Here's how the part is built. I have some questions about the finished solid (model axes, mm). Coordinates: 2 decimals unless noted, no trailing zeros. Loops run counter-clockwise (first coordinate to the right, second up) from the corner with the lowest first, then second, coordinate; pieces in that order, holes last. Notation, with made-up numbers: M 27.25,49.25 L 43.25,49.25 A24 ccw 43.25,88.25 Z; hole C -22.75,52.25 d11. An arc over 180 degrees is marked long. Use CSV: the item, a comma, the result in double quotes. Start each with the question number.
Q1. If we section it at D-D (y = 2.5): Please give me the cut outline in (x, z), and give its area (3 significant figures).
Q2. For pin 1 Ø5 at (y, z) = (2.5, 7.5) entering from +X; pin 2 Ø5 at (x, y) = (5, 4) entering from +Z, each with a flat end and sliding along its axis, tell me the tip position at first contact or that it passes through.
Q3. If we section it at C-C (x = 6): Please give me the cut outline in (y, z), and give its area (3 significant figures).
Q4. If we section it at B-B (y = -4): Please give me the cut outline in (x, z), and give its area (3 significant figures).
Q5. If we section it at A-A (z = 2.25): Please give me the cut outline in (x, y).
Q6. Please list where these lines run through material, in increasing order: probe 1 along Y at (x, z) = (7, 7); probe 2 along Y at (x, z) = (8.5, 1.75); probe 3 along X at (y, z) = (-2.5, 1). Write a range as [from, to].
from build123d import *

# Parameters (mm, degrees)
F0_W     = 19
F0_H     = 11
F1_DEPTH = 11
F3_DEPTH = 25
F4_R     = 5


with BuildPart() as f1:
    # F0 (on Top) → F1 (new body)
    with BuildSketch(Plane.XY):
        Rectangle(F0_W, F0_H)
    extrude(amount=F1_DEPTH)

    # F2 (on face) → F3 (cut)
    with BuildSketch(Plane.XZ.offset(5.5)):
        Polygon((-9.5, 11), (-9.5, 9), (9.5, 11), align=None)
    extrude(amount=-F3_DEPTH, mode=Mode.SUBTRACT)

    # F4
    f4_edges = [f1.edges().sort_by_distance(p)[0] for p in [
        (0, -5.5, 10),
        (9.5, 0, 11),
        (0, 5.5, 10),
        (9.5, -5.5, 5.5),
        (9.5, 5.5, 5.5),
    ]]
    fillet(f4_edges, radius=F4_R)


solid = f1.part
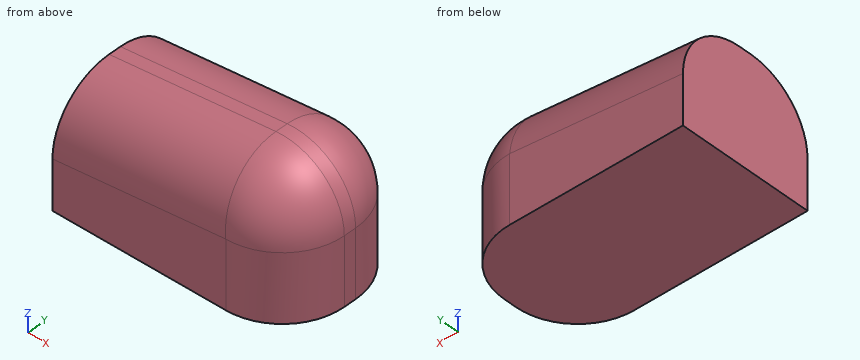
Results below:
1,outline,"M -9.5,0 L 9.08,0 L 9.08,5.45 A4.58 ccw 4.02,10 L -9.5,8.58 Z"
1,area,"172 mm^2"
2,pin 1,"x = 9.49"
2,pin 2,"z = 10.34"
3,outline,"M -5.27,0 L 5.27,0 L 5.27,5.45 A4.77 ccw 0.5,10.22 L -0.5,10.22 A4.77 ccw -5.27,5.45 Z"
3,area,"97.9 mm^2"
4,outline,"M -9.5,0 L 8.07,0 L 8.07,5.45 A3.57 ccw 4.13,9 L -9.5,7.56 Z"
4,area,"146 mm^2"
5,outline,"M -9.5,-5.5 L 4.5,-5.5 A5 ccw 9.5,-0.5 L 9.5,0.5 A5 ccw 4.5,5.5 L -9.5,5.5 Z"
6,probe 1,"[-4.54, 4.54]"
6,probe 2,"[-3.5, 3.5]"
6,probe 3,"[-9.5, 9.08]"
